```python
from build123d import *

# Parameters (mm, degrees)
F0_R      = 34.5
F1_DEPTH  = 15
F2_T      = -2.5
F3_R      = 42.5
F3_R_2    = 34.5
F4_DEPTH  = 2
F4_FACE_R = 42.5
F6_R      = 2.5
F8_R      = 1
F9_R      = 1


with BuildPart() as f1:
    # F0 (on Top) → F1 (new body)
    with BuildSketch(Plane.XY):
        Circle(F0_R)
    extrude(amount=F1_DEPTH)

    # F2
    f2_openings = [f1.faces().sort_by_distance(p)[0] for p in [
        (0, 0, 0),
    ]]
    offset(amount=F2_T, openings=f2_openings)

    # F3 (on face) → F4 (join)
    with BuildSketch(Plane.XY.offset(15)):
        Circle(F3_R)
        Circle(F3_R_2, mode=Mode.SUBTRACT)
        Circle(F3_R_2)
    extrude(amount=F4_DEPTH)

    # F4_face (on face) → F7 section 0
    with BuildSketch(Plane.XY.offset(17)):
        Circle(F4_FACE_R)
    # F6 (on offset) → F7 section 1
    with BuildSketch(Plane.XY.offset(19)):
        Circle(F6_R)
    loft()

    # F8
    f8_edges = [f1.edges().sort_by_distance(p)[0] for p in [
        (-42.5, 0, 17),
    ]]
    fillet(f8_edges, radius=F8_R)

    # F9
    f9_edges = [f1.edges().sort_by_distance(p)[0] for p in [
        (-42.5, 0, 15),
    ]]
    fillet(f9_edges, radius=F9_R)


solid = f1.part
```
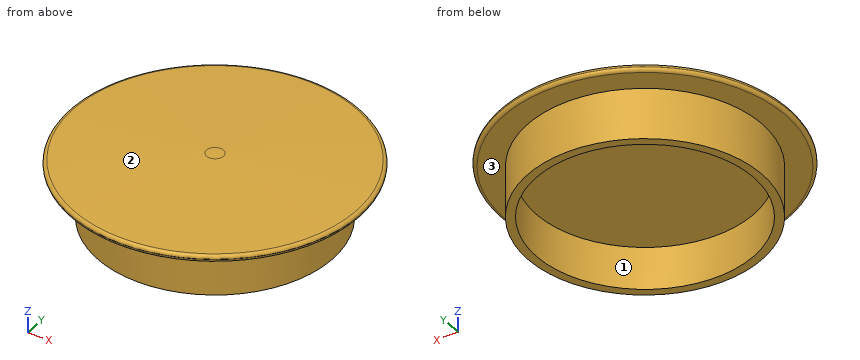
The model under review builds one solid part; all positions refer to its coordinate system, in mm. Face numbers are marked on the shaded views. Round coordinates to 2 decimals unless told otherwise and drop trailing zeros. Order: outer loops, then holes, each group sorted by start corner. A loop starts at its lowest first (then second) coordinate and runs counter-clockwise, first axis right, second up. Notation, with made-up numbers: (28, -1) -> (41, -1) arc R21 cw to (41, 15) -> close; hole circle Ø4 at (56, 28). An arc over 180 degrees is marked (long way). One line per item, written item: value. Start each with the question number.
Q1. Clearance check with flat-ended pins moving along their axes: pin 1 Ø4 at (x, y) = (1, 23.5) entering from -Z; pin 2 Ø5 at (x, z) = (30.5, 6.5) entering from +Y; pin 3 Ø8 at (y, z) = (-15.5, 13) entering from +X. State where each tip first meets the part, or that it passes through.
Q2. Mouldability with a two-part tool opening along Y and no side actions: class the marked faces 1, 2 and 3 as released by +Y, released by -Y, zero draft, split by the parting line, or undercut.
Q3. Wall thickness on line 1 (Y direction, x = 0, z = 8); line 2 (Y direction, x = 9.5, z = 11.25); line 3 (X direction, y = 17, z = 5.5): over which ranges is each line inside the solid? List them lowest first.
Q4. Take a section at A-A (z = 3.75). Write out the cut boundary in (x, y).
Reported:
1. pin 1: stops at z = 12.5
1. pin 2: stops at y = 20.16
1. pin 3: stops at x = 40.56
2. face 1: undercut
2. face 2: split by the parting line
2. face 3: zero draft
3. line 1: y = -34.5 to -32, 32 to 34.5
3. line 2: y = -33.17 to -30.56, 30.56 to 33.17
3. line 3: x = -30.02 to -27.11, 27.11 to 30.02
4. outline: circle Ø69 at (0, 0); hole circle Ø64 at (0, 0)
